The model under review builds one solid part; all positions refer to its coordinate system, in mm. A direction names the side the tool comes from. Coordinates: 2 decimals unless noted, no trailing zeros. Write each loop counter-clockwise with the first axis right and the second up, starting at its lowest first coordinate (ties: lowest second). Pieces come first, ordered by that corner, then holes.
1) Add section B-B, the plane y = 0. State the section outline as (x, z) points, then the cut area to 3 significant figures.
2) For line 1 (Y direction, x = 31, z = 27); line 2 (Y direction, x = 35, z = 89); line 3 (Y direction, x = -12.5, z = 15), list the stretches that pass through material, from the lowest coordinate up.
3) For P1, Ø3, axis at x = -0.5, y = 28, coming from the +Z side; P2, Ø5, axis at y = 54, z = 12, coming from the -X side; P3, Ø8, axis at x = -22, z = 42.5, coming from the -Y side, all flat-tipped, find the tip position at first contact; note any pin that passes through.
4) Machinability: for faces 1 (the conical face through (49.136, 0.737, 33.525)), 2 (the flat face through (61.976, 0, 20)), 3 (the conical face through (-49.59, 0.733, 33.325)), which of the approach directions +Z, -Z, +X, -X, +Y, -Y give a long, thin tool a straight path to every point of the face, cutting with its end or side? Answer none if there is none.
5) Add section A-A, the plane x = 40. State the section outline as (y, z) points.
6) Add section C-C, the plane x = -32. State the section outline as (y, z) points.
7) Mouldability with a two-part tool opening along Y and no side actions: class faces 4 (the cylindrical face through (-0.599, 2.394, 108.846)), 5 (the flat face through (-42.764, 8, 99)), 6 (the conical face through (30.37, 2.07, 93.91)) as released by +Y, released by -Y, zero draft, split by the parting line, or undercut.
from build123d import *

# Parameters (mm, degrees)
REVOLVE_1_ANGLE = 180


with BuildPart() as part:
    # 草图1 → 旋转1 (revolve)
    with BuildSketch(Plane.XY):
        Polygon((-61.976468087, 19.212705107), (61.976468087, 19.212705107), (61.976468087, 27.889410639), (29.542116455, 42.143998299), (29.542116455, 93.584466811), (42.76376298, 99.162348939), (42.76376298, 108.871995605), (-42.76376298, 108.871995605), (-42.76376298, 99.162348939), (-29.542116455, 93.584466811), (-29.542116455, 42.143998299), (-61.976468087, 27.889410639), align=None)
    revolve(axis=Axis((0, 0, 0), (1, 0, 0)), revolution_arc=REVOLVE_1_ANGLE)


solid = part.part
Geometry results:
1. outline: (-61.98, 19.21) - (61.98, 19.21) - (61.98, 27.89) - (29.54, 42.14) - (29.54, 93.58) - (42.76, 99.16) - (42.76, 108.87) - (-42.76, 108.87) - (-42.76, 99.16) - (-29.54, 93.58) - (-29.54, 42.14) - (-61.98, 27.89) - close
1. area: 6,650 mm2
2. line 1: y = -105.47 to -90.25, -31.52 to 31.52, 90.25 to 105.47
2. line 2: y = -62.71 to -35.68, 35.68 to 62.71
2. line 3: y = -107.83 to -12.01, 12.01 to 107.83
3. P1: stops at z = 105.6
3. P2: stops at x = -29.54
3. P3: stops at y = -101.84
4. face 1: +X
4. face 2: +Z, -Z, +X, +Y, -Y
4. face 3: -X
5. outline: (-108.87, 0) - (-98, 0) arc R98 cw to (98, 0) - (108.87, 0) arc R108.87 ccw to start; (-37.55, 0) - (-19.21, 0) arc R19.21 cw to (19.21, 0) - (37.55, 0) arc R37.55 ccw to start
6. outline: (-108.87, 0) - (-94.62, 0) arc R94.62 cw to (94.62, 0) - (108.87, 0) arc R108.87 ccw to start; (-41.06, 0) - (-19.21, 0) arc R19.21 cw to (19.21, 0) - (41.06, 0) arc R41.06 ccw to start
7. face 4: split by the parting line
7. face 5: zero draft
7. face 6: undercut
